from build123d import *

# Parameters (mm, degrees)
F0_R     = 9.525
F1_DEPTH = 6.35


with BuildPart() as f1:
    # F0 (on Top) → F1 (new body)
    with BuildSketch(Plane.XY):
        with BuildLine():
            Line((104.954476, 56.91301), (16.054476, 56.91301))
            ThreePointArc((16.054476, 56.91301), (4.559189, 50.466038), (0, 38.1))
            Line((0, 38.1), (0, 15.24))
            Line((0, 15.24), (28.189888, 15.24))
            ThreePointArc((28.189888, 15.24), (43.144494, 26.272727), (61.066383, 31.188743))
            ThreePointArc((61.066383, 31.188743), (64.084666, 31.724007), (67.12522, 31.334683))
            ThreePointArc((67.12522, 31.334683), (72.442024, 27.683294), (74.48932, 21.566953))
            Line((74.48932, 21.566953), (125.122593, 21.566953))
            Line((125.122593, 21.566953), (125.122593, -21.566953))
            Line((125.122593, -21.566953), (74.48932, -21.566953))
            ThreePointArc((74.48932, -21.566953), (72.442024, -27.683294), (67.12522, -31.334683))
            ThreePointArc((67.12522, -31.334683), (64.084666, -31.724007), (61.066383, -31.188743))
            ThreePointArc((61.066383, -31.188743), (43.144494, -26.272727), (28.189888, -15.24))
            Line((28.189888, -15.24), (0, -15.24))
            Line((0, -15.24), (0, -38.1))
            ThreePointArc((0, -38.1), (4.559189, -50.466038), (16.054476, -56.91301))
            Line((16.054476, -56.91301), (104.954476, -56.91301))
            Line((104.954476, -56.91301), (144.209702, -46.394604))
            Line((144.209702, -46.394604), (148.998593, -38.1))
            Line((148.998593, -38.1), (148.998593, 0))
            Line((148.998593, 0), (148.998593, 38.1))
            Line((148.998593, 38.1), (144.209702, 46.394604))
            Line((144.209702, 46.394604), (104.954476, 56.91301))
        make_face()
        with Locations((19.05, -38.1)):
            Circle(F0_R, mode=Mode.SUBTRACT)
        with Locations((104.954476, -38.4048)):
            Circle(F0_R, mode=Mode.SUBTRACT)
        with Locations((19.05, 38.1)):
            Circle(F0_R, mode=Mode.SUBTRACT)
        with Locations((104.954476, 38.4048)):
            Circle(F0_R, mode=Mode.SUBTRACT)
        with BuildLine():
            ThreePointArc((67.12522, 31.334683), (64.084666, 31.724007), (61.066383, 31.188743))
            ThreePointArc((61.066383, 31.188743), (64.093623, 31.352148), (67.12522, 31.334683))
        make_face()
        with BuildLine():
            ThreePointArc((61.066383, -31.188743), (64.084666, -31.724007), (67.12522, -31.334683))
            ThreePointArc((67.12522, -31.334683), (64.093623, -31.352148), (61.066383, -31.188743))
        make_face()
    extrude(amount=F1_DEPTH)


solid = f1.part
Model file for the job. Use its own axes, mm. A direction names the side the tool comes from. Round coordinates to 2 decimals unless told otherwise and drop trailing zeros. Order: outer loops, then holes, each group sorted by start corner. A loop starts at its lowest first (then second) coordinate and runs counter-clockwise, first axis right, second up.
(1) Band-saw the part on A-A (x = 19.05). List the corners of the cut face in (y, z) (3 decimals), then the cut area to 3 significant figures.
(2) Band-saw the part on D-D (y = -42). List the corners of the cut face in (x, z).
(3) 3-axis set-ups, long thin cutter, end or side, ignore diameter. For faces 4 (the face through (14, -15.24, 3)), 5 (the face through (148.999, -1, 3)), 6 (the face through (64.05, 31.35, 3.13)): which of +Z, -Z, +X, -X, +Y, -Y reach the whole face in a straight line?
(4) Band-saw the part on C-C (z = 4.5). List the corners of the cut face in (x, y) (3 decimals).
(5) Pin check, flat tips, straight feed: pin 1 (1.5 mm diameter, centred on x = 116, z = 5.5, fed in from +Y); pin 2 (3 mm diameter, centred on x = 11, z = 3, fed in from +Y); pin 3 (1.5 mm diameter, centred on y = -13, z = 1.5, fed in from -X). Stop position of each tip, or through.
(6) Drill centre lines: line 1 (Y direction, x = 19, z = 2); line 2 (X direction, y = 42.5, z = 6); line 3 (Y direction, x = 94, z = 3.5). Where is each one in solid material? Low to high.
(7) Pull direction X, two halves, no side cores. Call faces 1 (the face through (125.123, 0, 3)), 2 (the face through (90, 26, 0)), 3 (the face through (124.307, -51.727, 3.131)): released by +X, released by -X, zero draft, split by the parting line, or undercut.
(8) Band-saw the part on B-B (y = 27). List the corners of the cut face in (x, z), then the cut area to 3 significant figures.
Verdict:
1. outline: (-56.913, 0) - (-47.625, 0) - (-47.625, 6.35) - (-56.913, 6.35) - close; (-28.575, 0) - (-15.24, 0) - (-15.24, 6.35) - (-28.575, 6.35) - close; (15.24, 0) - (28.575, 0) - (28.575, 6.35) - (15.24, 6.35) - close; (47.625, 0) - (56.913, 0) - (56.913, 6.35) - (47.625, 6.35) - close
1. area: 287 mm2
2. outline: (0.4, 0) - (10.36, 0) - (10.36, 6.35) - (0.4, 6.35) - close; (27.74, 0) - (96.13, 0) - (96.13, 6.35) - (27.74, 6.35) - close; (113.77, 0) - (146.75, 0) - (146.75, 6.35) - (113.77, 6.35) - close
3. face 4: +Z, -Z, -X
3. face 5: +Z, -Z, +X, +Y, -Y
3. face 6: +Z, -Z
4. outline: (0, -38.1) arc R19.05 ccw to (16.054, -56.913) - (104.954, -56.913) - (144.21, -46.395) - (148.999, -38.1) - (148.999, 38.1) - (144.21, 46.395) - (104.954, 56.913) - (16.054, 56.913) arc R19.05 ccw to (0, 38.1) - (0, 15.24) - (28.19, 15.24) arc R50.8 cw to (61.066, 31.189) arc R50.8 cw to (67.125, 31.335) arc R10.16 cw to (74.489, 21.567) - (125.123, 21.567) - (125.123, -21.567) - (74.489, -21.567) arc R10.16 cw to (67.125, -31.335) arc R50.8 cw to (61.066, -31.189) arc R50.8 cw to (28.19, -15.24) - (0, -15.24) - close; hole circle Ø19.05 at (19.05, -38.1); hole circle Ø19.05 at (19.05, 38.1); hole circle Ø19.05 at (104.954, -38.405); hole circle Ø19.05 at (104.954, 38.405)
5. pin 1: stops at y = 54.15
5. pin 2: stops at y = 55.99
5. pin 3: stops at x = 125.12
6. line 1: y = -56.91 to -47.62, -28.58 to -15.24, 15.24 to 28.58, 47.62 to 56.91
6. line 2: x = 0.52 to 10.6, 27.5 to 96.35, 113.55 to 146.46
6. line 3: y = -56.91 to -21.57, 21.57 to 56.91
7. face 1: undercut
7. face 2: zero draft
7. face 3: released by +X
8. outline: (0, 0) - (44.71, 0) - (44.71, 6.35) - (0, 6.35) - close; (72.91, 0) - (149, 0) - (149, 6.35) - (72.91, 6.35) - close
8. area: 767 mm2
